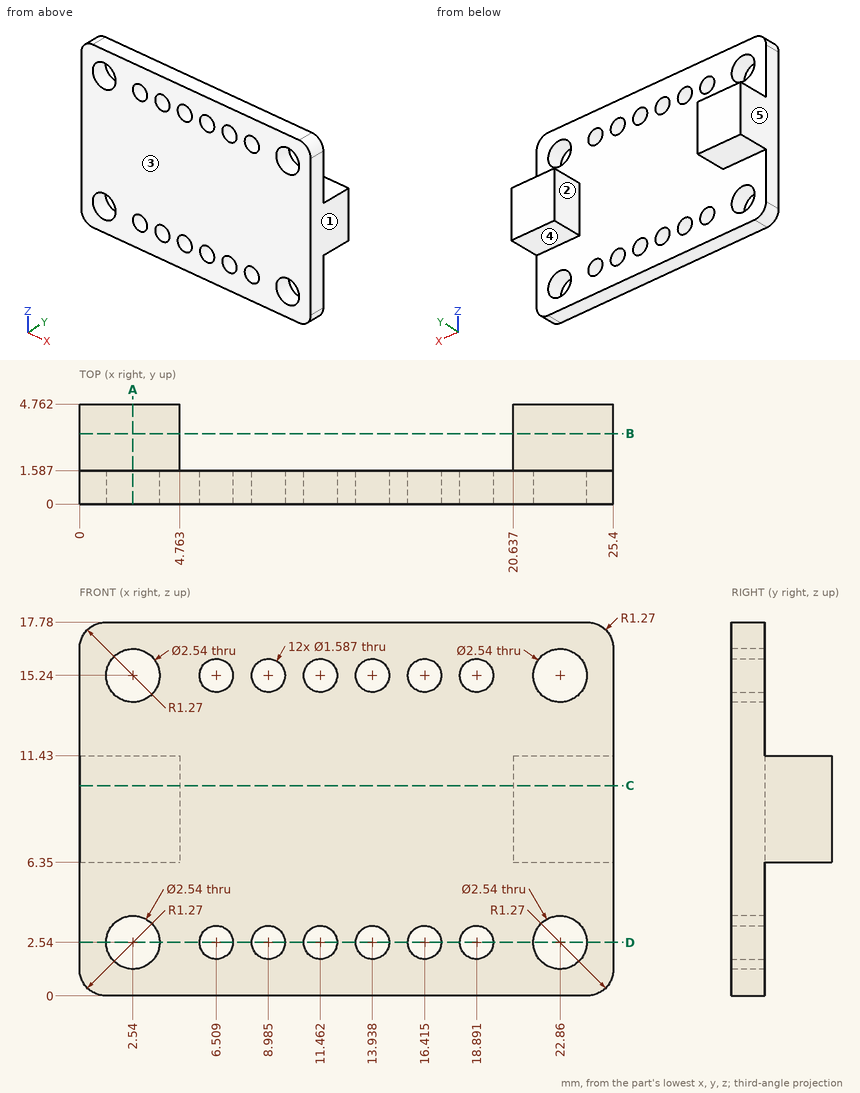
Answer from the drawing. Dimensions are ordinates in mm from the lowest x, y and z of the part. A direction names the side the tool comes from. Give positions to 0.01 mm unless a question says otherwise; leave off trailing zeros. Order: outer loops, then holes, each group sorted by start corner. A loop starts at its lowest first (then second) coordinate and runs counter-clockwise, first axis right, second up. Notation, with made-up numbers: (-0.75, 56) - (13.25, 56) arc R27 cw to (13.25, 82) - close; hole circle Ø10 at (-13, -14.75). An arc over 180 degrees is marked (long way). One line per item, written item: value. Start each with the question number.
1) A tool of negligible diameter and unlimited length cuts with its end or side. For the marked faces 4 and 5, from which of +Z, -Z, +X, -X, +Y, -Y can it reach the whole face along a straight path? Write none if from no direction.
2) A cutting plane is placed at A-A on x = 2.54. Give the vertices of the cut face in (y, z).
3) The mould has two halves that part along X. Classify the marked faces 1, 2 and 3: released by +X, released by -X, zero draft, split by the parting line, or undercut.
4) A cutting plane is placed at D-D on z = 2.54. State how many separate pieces and enclosed holes the cut face has.
5) A cutting plane is placed at C-C on z = 10. Give the vertices of the cut face in (x, y).
6) Given pin 1 Ø1.8 at (x, z) = (16.41, 2.54) entering from +Y; pin 2 Ø1 at (x, y) = (2.5, 3) entering from +Z; pin 3 Ø6 at (x, z) = (22, 11.5) entering from -Y; pin 4 Ø2.5 at (x, y) = (23.5, 3) entering from -Z, each flat-ended and moving along its own axis, determine where each tip first touches the part or whether it passes through.
7) Find the intervals of material crossed by L1, parallel to Z at x = 2.54, y = 1.2; L2, parallel to Z at x = 19.5, y = 1.1; L3, parallel to X at y = 0.65, z = 3.5, in increasing order.
8) A cutting plane is placed at B-B on y = 3.35. Give the vertices of the cut face in (x, z).
Answer sheet:
1. face 4: -Z, +X, -X, +Y
1. face 5: +Z, -Z, -X, +Y, -Y
2. outline: (0, 0) - (1.59, 0) - (1.59, 1.27) - (0, 1.27) - close; (0, 3.81) - (1.59, 3.81) - (1.59, 6.35) - (4.76, 6.35) - (4.76, 11.43) - (1.59, 11.43) - (1.59, 13.97) - (0, 13.97) - close; (0, 16.51) - (1.59, 16.51) - (1.59, 17.78) - (0, 17.78) - close
3. face 1: released by +X
3. face 2: undercut
3. face 3: zero draft
4. separate pieces: 9
4. enclosed holes: 0
5. outline: (0, 0) - (25.4, 0) - (25.4, 4.76) - (20.64, 4.76) - (20.64, 1.59) - (4.76, 1.59) - (4.76, 4.76) - (0, 4.76) - close
6. pin 1: stops at y = 1.59
6. pin 2: stops at z = 11.43
6. pin 3: stops at y = 0
6. pin 4: stops at z = 6.35
7. L1: z = 0 to 1.27, 3.81 to 13.97, 16.51 to 17.78
7. L2: z = 0 to 2.03, 3.05 to 14.73, 15.75 to 17.78
7. L3: x = 0 to 1.71, 3.37 to 22.03, 23.69 to 25.4
8. outline: (0, 6.35) - (4.76, 6.35) - (4.76, 11.43) - (0, 11.43) - close; (20.64, 6.35) - (25.4, 6.35) - (25.4, 11.43) - (20.64, 11.43) - close
